Can you work these out from the model? Positions are in its coordinate system, mm. A direction names the side the tool comes from. Give positions to 0.01 mm unless a question says otherwise; leave off trailing zeros. Write each loop counter-clockwise with the first axis right and the second up, starting at its lowest first coordinate (ties: lowest second). Pieces come first, ordered by that corner, then holes. Notation, with made-up numbers: (69, 71) -> (109, 71) arc R24 cw to (109, 100) -> close; hole circle Ø1 at (53.25, 5.5). An arc over 180 degrees is marked (long way). Answer as CSV lines item,"result". Start each with the question number.
1. On a 3-axis mill with a long thin cutter (end or side, diameter ignored), from which of +Z, -Z, +X, -X, +Y, -Y can I reach the whole of each face in a straight line? I mean faces 1 (the face through (1, 0, 8)), 2 (the face through (-7, 1, 3)). Say none if no direction works.
2. If we section it at A-A on y = -2.25: Write out the boundary of the cut face in (x, z).
3. I'm going to push a flat-ended pin straight in: P1, Ø1.9, axis at x = 0, y = 3, coming from the -Z side. Where does the tip first touch, or does it pass through?
4. I need wall thicknesses on line 1 (Y direction, x = 0, z = 2); line 2 (Y direction, x = 0, z = 3.25); line 3 (Z direction, x = -6.25, y = 4.5). Which ranges of each line are inside material? Lowest first, please. Write a range as [from, to].
5. If we mould it in two halves opening along X, with no side actions, what happens to faces 3 (the face through (0, 0, 0)), 4 (the face through (-6, 0, 5)), 5 (the face through (0.336, -1.487, 4.056)), 6 (the face through (-0.336, 1.487, 4.056))? For each: pulls with the +X half, pulls with the -X half, needs draft (parallel to the pull), parting line crosses it, or undercut.
6. If we section it at C-C on x = 0: Write out the boundary of the cut face in (y, z).
7. If we section it at B-B on z = 6: Write out the boundary of the cut face in (x, y).
8. If we section it at D-D on y = 0: Write out the boundary of the cut face in (x, z).
```python
from build123d import *

# Parameters (mm, degrees)
SKETCH1_R           = 10
BOSS_EXTRUDE1_DEPTH = 3
SKETCH2_R           = 7.5
BOSS_EXTRUDE2_DEPTH = 5
SKETCH3_R           = 1.55
CUT_EXTRUDE1_DEPTH  = 17.248076809


with BuildPart() as part:
    # Sketch1 → Boss-Extrude1 (new body)
    with BuildSketch(Plane.XY):
        Circle(SKETCH1_R)
    extrude(amount=BOSS_EXTRUDE1_DEPTH)

    # Sketch2 → Boss-Extrude2 (add)
    with BuildSketch(Plane.XY.offset(3)):
        with Locations((1.5, 0)):
            Circle(SKETCH2_R)
    extrude(amount=BOSS_EXTRUDE2_DEPTH)

    # Sketch3 → Cut-Extrude1 (cut, through all)
    with BuildSketch(Plane.XY.offset(8)):
        with Locations((0, 3)):
            Circle(SKETCH3_R)
        with Locations(Location((0, -3, 0), (0, 0, 180))):
            Circle(SKETCH3_R)
    extrude(amount=-CUT_EXTRUDE1_DEPTH, mode=Mode.SUBTRACT)


solid = part.part
```
Computed values:
1,face 1,"+Z, +X, -X, +Y, -Y"
1,face 2,"+Z"
2,outline,"(-9.74, 0) -> (-1.36, 0) -> (-1.36, 8) -> (-5.65, 8) -> (-5.65, 3) -> (-9.74, 3) -> close; (1.36, 0) -> (9.74, 0) -> (9.74, 3) -> (8.65, 3) -> (8.65, 8) -> (1.36, 8) -> close"
3,P1,"passes through"
4,line 1,"y = [-10, -4.55], [-1.45, 1.45], [4.55, 10]"
4,line 2,"y = [-7.35, -4.55], [-1.45, 1.45], [4.55, 7.35]"
4,line 3,"z = [0, 3]"
5,face 3,"needs draft"
5,face 4,"parting line crosses it"
5,face 5,"undercut"
5,face 6,"undercut"
6,outline,"(-10, 0) -> (-4.55, 0) -> (-4.55, 8) -> (-7.35, 8) -> (-7.35, 3) -> (-10, 3) -> close; (-1.45, 0) -> (1.45, 0) -> (1.45, 8) -> (-1.45, 8) -> close; (4.55, 0) -> (10, 0) -> (10, 3) -> (7.35, 3) -> (7.35, 8) -> (4.55, 8) -> close"
7,outline,"circle Ø15 at (1.5, 0); hole circle Ø3.1 at (0, -3); hole circle Ø3.1 at (0, 3)"
8,outline,"(-10, 0) -> (10, 0) -> (10, 3) -> (9, 3) -> (9, 8) -> (-6, 8) -> (-6, 3) -> (-10, 3) -> close"
